from build123d import *

# Parameters (mm, degrees)
F0_W     = 166
F0_H     = 81
F0_W_2   = 150
F0_H_2   = 63.2
F0_R     = 1.75
F0_W_3   = 98.5
F0_H_3   = 40.7
F0_W_4   = 6
F0_H_4   = 6
F0_W_5   = 13
F0_H_5   = 12
F0_R_2   = 3.75
F0_R_3   = 2.25
F1_DEPTH = 3


with BuildPart() as f1:
    # F0 (on Top) → F1 (new body)
    with BuildSketch(Plane.XY):
        Rectangle(F0_W, F0_H)
        Rectangle(F0_W_2, F0_H_2, mode=Mode.SUBTRACT)
        Rectangle(F0_W_2, F0_H_2)
        with Locations((-72.38, -20.78)):
            Circle(F0_R, mode=Mode.SUBTRACT)
        with Locations((-12.75, -1.75)):
            Rectangle(F0_W_3, F0_H_3, mode=Mode.SUBTRACT)
        with Locations((72.38, -20.78)):
            Circle(F0_R, mode=Mode.SUBTRACT)
        with Locations((62.5, -15.9)):
            Rectangle(F0_W_4, F0_H_4, mode=Mode.SUBTRACT)
        with Locations((-72.38, 28.98)):
            Circle(F0_R, mode=Mode.SUBTRACT)
        with Locations((62.5, 2.1)):
            Rectangle(F0_W_5, F0_H_5, mode=Mode.SUBTRACT)
        with Locations((72.38, 28.98)):
            Circle(F0_R, mode=Mode.SUBTRACT)
        with Locations((62.5, 2.1)):
            Rectangle(F0_W_5, F0_H_5)
        with Locations((62.5, 2.1)):
            Circle(F0_R_2, mode=Mode.SUBTRACT)
        with Locations((62.5, -15.9)):
            Rectangle(F0_W_4, F0_H_4)
        with Locations((62.5, -15.9)):
            Circle(F0_R_3, mode=Mode.SUBTRACT)
    extrude(amount=F1_DEPTH)


solid = f1.part
CAD build for the part. Positions are in the model's coordinates, mm. A direction names the side the tool comes from. Coordinates: 2 decimals unless noted, no trailing zeros. Write each loop counter-clockwise with the first axis right and the second up, starting at its lowest first coordinate (ties: lowest second). Pieces come first, ordered by that corner, then holes. Notation, with made-up numbers: M -37,51.25 L 8,51.25 A26 cw 8,80.25 Z; hole C 20.25,-21.5 d8. An arc over 180 degrees is marked long. Return JSON: item names as keys, results as strings.
Item 1: Slice it at D-D, the plane z = 0.7. Write the cut outline in (x, y), and give its area (3 significant figures).
Findings below:
{"outline": "M -83,-40.5 L 83,-40.5 L 83,40.5 L -83,40.5 Z; hole C -72.38,-20.78 d3.5; hole C -72.38,28.98 d3.5; hole M -62,-22.1 L 36.5,-22.1 L 36.5,18.6 L -62,18.6 Z; hole C 62.5,2.1 d7.5; hole C 62.5,-15.9 d4.5; hole C 72.38,-20.78 d3.5; hole C 72.38,28.98 d3.5", "area": "9,340 mm2"}
Item 2: Slice it at A-A, the plane y = 28.98. Write the cut outline in (x, z), and give its area (3 significant figures).
Findings below:
{"outline": "M -83,0 L -74.13,0 L -74.13,3 L -83,3 Z; M -70.63,0 L 70.63,0 L 70.63,3 L -70.63,3 Z; M 74.13,0 L 83,0 L 83,3 L 74.13,3 Z", "area": "477 mm2"}
Item 3: Slice it at B-B, the plane x = -72.38. Write the cut outline in (y, z), and give its area (3 significant figures).
Findings below:
{"outline": "M -40.5,0 L -22.53,0 L -22.53,3 L -40.5,3 Z; M -19.03,0 L 27.23,0 L 27.23,3 L -19.03,3 Z; M 30.73,0 L 40.5,0 L 40.5,3 L 30.73,3 Z", "area": "222 mm2"}
Item 4: Two-plate mould, pull along X, no slides. Class faces 1 (the flat face through (-13, 18.6, 1)), 2 (the flat face through (-1, -26, 3)), 3 (the cylindrical face through (-70.711, -20.254, 1.479)), 4 (the flat face through (-83, -1, 1)): +X half, -X half, draft (parallel to the pull), parting line (faces both ways), or undercut.
Findings below:
{"face 1": "undercut", "face 2": "draft", "face 3": "undercut", "face 4": "-X half"}
Item 5: Slice it at C-C, the plane x = -49.5. Write the cut outline in (y, z).
Findings below:
{"outline": "M -40.5,0 L -22.1,0 L -22.1,3 L -40.5,3 Z; M 18.6,0 L 40.5,0 L 40.5,3 L 18.6,3 Z"}
Item 6: Probe line 1 (Y direction, x = 72.38, z = 1.8); line 2 (Y direction, x = 62.5, z = 0.95); line 3 (X direction, y = 2.5, z = 1.3). List the from-to ranges inside material, lowest first. Write a range as from..to.
Findings below:
{"line 1": "y = -40.5..-22.53, -19.03..27.23, 30.73..40.5", "line 2": "y = -40.5..-18.15, -13.65..-1.65, 5.85..40.5", "line 3": "x = -83..-62, 36.5..58.77, 66.23..83"}
Item 7: Which spindle directions (+Z, -Z, +X, -X, +Y, -Y) get a long thin tool onto all of the face, cutting with end or side? Do faces 5 (the flat face through (-13, -22.1, 1)), 6 (the flat face through (-1, -26, 0)). Say none if no direction does.
Findings below:
{"face 5": "+Z, -Z", "face 6": "-Z, +X, -X, +Y, -Y"}
